Source: CAD feature listing. Evaluate the final solid. Frame: model axes, mm. Face numbers are marked on the shaded views. A direction names the side the tool comes from. Coordinates: 2 decimals unless noted, no trailing zeros. Order: outer loops, then holes, each group sorted by start corner. A loop starts at its lowest first (then second) coordinate and runs counter-clockwise, first axis right, second up. Notation, with made-up numbers: (-27.75, 3) -> (30.25, 3) arc R26 cw to (30.25, 20) -> close; hole circle Ø6 at (38, -10.5). An arc over 180 degrees is marked (long way). Put each result on its own line as item: value.
from build123d import *

# Parameters (mm, degrees)
F0_W     = 30
F0_H     = 45
F1_DEPTH = 5
F2_R     = 3.087688
F3_DEPTH = 5
F4_R     = 5.921375
F5_DEPTH = 1.6
F6_R     = 1.75
F7_DEPTH = 5


with BuildPart() as f1:
    # F0 (on Top) → F1 (new body)
    with BuildSketch(Plane.XY):
        Rectangle(F0_W, F0_H)
    extrude(amount=F1_DEPTH)

    # F2 (on face) → F3 (cut, through all)
    with BuildSketch(Plane.XY.offset(5)):
        with Locations((-7.5, 10)):
            Circle(F2_R)
        with Locations((-7.5, -5)):
            Circle(F2_R)
        with Locations((7.5, 10)):
            Circle(F2_R)
        with Locations((7.5, -5)):
            Circle(F2_R)
    extrude(amount=-F3_DEPTH, mode=Mode.SUBTRACT)

    # F4 (on face) → F5 (cut)
    with BuildSketch(Plane.XY.offset(5)):
        with Locations((-7.5, 10)):
            Circle(F4_R)
        with Locations((7.5, 10)):
            Circle(F4_R)
        with Locations((7.5, -5)):
            Circle(F4_R)
        with Locations((-7.5, -5)):
            Circle(F4_R)
    extrude(amount=-F5_DEPTH, mode=Mode.SUBTRACT)

    # F6 (on face) → F7 (cut, through all)
    with BuildSketch(Plane.XY.offset(5)):
        with Locations((5, 19.5)):
            Circle(F6_R)
        with Locations((-2.5, -19.5)):
            Circle(F6_R)
    extrude(amount=-F7_DEPTH, mode=Mode.SUBTRACT)


solid = f1.part
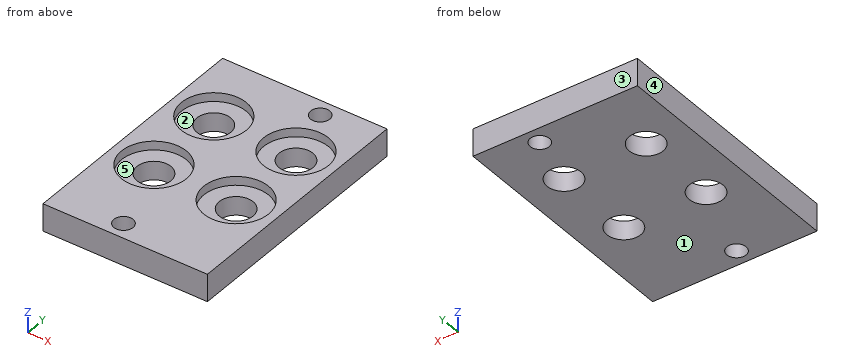
1. Cut plane C-C on y = -19.5. Output: boundary loops of the cut face in (x, z), plus the area to 4 significant figures.
Numbers:
outline: (-15, 0) -> (-4.25, 0) -> (-4.25, 5) -> (-15, 5) -> close; (-0.75, 0) -> (15, 0) -> (15, 5) -> (-0.75, 5) -> close
area: 132.5 mm2
2. Cut plane B-B on y = 10. Output: boundary loops of the cut face in (x, z), plus the area to 3 significant figures.
Numbers:
outline: (-15, 0) -> (-10.59, 0) -> (-10.59, 3.4) -> (-13.42, 3.4) -> (-13.42, 5) -> (-15, 5) -> close; (-4.41, 0) -> (4.41, 0) -> (4.41, 3.4) -> (1.58, 3.4) -> (1.58, 5) -> (-1.58, 5) -> (-1.58, 3.4) -> (-4.41, 3.4) -> close; (10.59, 0) -> (15, 0) -> (15, 5) -> (13.42, 5) -> (13.42, 3.4) -> (10.59, 3.4) -> close
area: 70.1 mm2
3. Cut plane D-D on z = 0.95. Output: boundary loops of the cut face in (x, y).
Numbers:
outline: (-15, -22.5) -> (15, -22.5) -> (15, 22.5) -> (-15, 22.5) -> close; hole circle Ø6.18 at (-7.5, -5); hole circle Ø6.18 at (-7.5, 10); hole circle Ø3.5 at (-2.5, -19.5); hole circle Ø3.5 at (5, 19.5); hole circle Ø6.18 at (7.5, -5); hole circle Ø6.18 at (7.5, 10)
4. First-contact query: pin 1 (3.5 mm diameter, centred on x = -7.5, y = 11.5, fed in from +Z). Flat tip, straight axial feed; report the tip coordinate or a pass-through.
Numbers:
pin 1: stops at z = 3.4
5. Cut plane A-A on x = -7.5. Output: boundary loops of the cut face in (y, z).
Numbers:
outline: (-22.5, 0) -> (-8.09, 0) -> (-8.09, 3.4) -> (-10.92, 3.4) -> (-10.92, 5) -> (-22.5, 5) -> close; (-1.91, 0) -> (6.91, 0) -> (6.91, 3.4) -> (4.08, 3.4) -> (4.08, 5) -> (0.92, 5) -> (0.92, 3.4) -> (-1.91, 3.4) -> close; (13.09, 0) -> (22.5, 0) -> (22.5, 5) -> (15.92, 5) -> (15.92, 3.4) -> (13.09, 3.4) -> close
6. Set-up query: the marked faces 4 and 5. Return all of +Z, -Z, +X, -X, +Y, -Y with unobstructed straight access to the full face (end or side cutting, diameter ignored); none if empty.
Numbers:
face 4: +Z, -Z, -X, +Y, -Y
face 5: +Z
7. Ray query, line 1 along Y through (x, z) = (7.5, 2.15); line 2 along Y through (x, z) = (-7.5, 4.55); line 3 along Y through (x, z) = (-2.5, 3.5). Return the intervals inside material, ascending.
Numbers:
line 1: y = -22.5 to -8.09, -1.91 to 6.91, 13.09 to 22.5
line 2: y = -22.5 to -10.92, 0.92 to 4.08, 15.92 to 22.5
line 3: y = -22.5 to -21.25, -17.75 to -8.17, -1.83 to 6.83, 13.17 to 22.5
8. Pull-direction query (Y, two-part tool) for the marked faces 1, 2 and 3; classes: pulls with the +Y half, pulls with the -Y half, needs draft (parallel to the pull), parting line crosses it, or undercut.
Numbers:
face 1: needs draft
face 2: undercut
face 3: pulls with the +Y half
